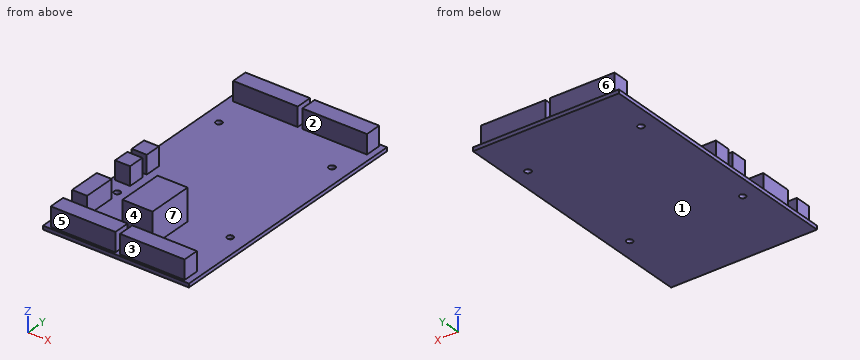
Autodesk Inventor part; units mm, degrees
ref_plane "YZ Plane" through (0, 0, 0) normal (1, 0, 0) x (0, 1, 0)
ref_plane "XZ Plane" through (0, 0, 0) normal (0, 1, 0) x (-1, 0, 0)
ref_plane "XY Plane" through (0, 0, 0) normal (0, 0, 1) x (1, 0, 0)
sketch "Sketch1" plane through (0, 0, 0) normal (0, 0, 1) x (1, 0, 0)
  line L0 (0, 0) -> (63.23, 0)
  line L1 (63.23, 0) -> (63.23, 113)
  line L2 (63.23, 113) -> (0, 113)
  line L3 (0, 113) -> (0, 0)
  line L4 (7.115, 91) -> (56.115, 91) construction
  line L5 (56.115, 91) -> (56.115, 33) construction
  line L6 (56.115, 33) -> (7.115, 33) construction
  line L7 (7.115, 33) -> (7.115, 91) construction
  circle A0 centre (7.115, 91) radius 1.35
  circle A1 centre (56.115, 91) radius 1.35
  circle A2 centre (56.115, 33) radius 1.35
  circle A3 centre (7.115, 33) radius 1.35
  point P0 (31.615, 91)
  point P1 (31.615, 113)
  dimension "d0" = 63.23
  dimension "d1" = 113
  dimension "d2" = 49
  dimension "d3" = 58
  dimension "d4" = 2.7
  dimension "d5" = 22
extrude "Extrusion1" add sketch "Sketch1" along normal blind 1.6
sketch "Sketch2" plane through (0, 0, 1.6) normal (0, 0, 1) x (1, 0, 0)
  point P0 (0, 0)
sketch "Sketch3" plane through (0, 0, 1.6) normal (0, 0, 1) x (1, 0, 0)
  line L0 (2.615, 112) -> (30.615, 112)
  line L1 (30.615, 112) -> (30.615, 105)
  line L2 (30.615, 105) -> (2.615, 105)
  line L3 (2.615, 105) -> (2.615, 112)
  line L4 (32.615, 112) -> (60.615, 112)
  line L5 (60.615, 112) -> (60.615, 105)
  line L6 (60.615, 105) -> (32.615, 105)
  line L7 (32.615, 105) -> (32.615, 112)
  line L8 (2.615, 1) -> (30.615, 1)
  line L9 (30.615, 1) -> (30.615, 8)
  line L10 (30.615, 8) -> (2.615, 8)
  line L11 (2.615, 8) -> (2.615, 1)
  line L12 (32.615, 1) -> (60.615, 1)
  line L13 (60.615, 1) -> (60.615, 8)
  line L14 (60.615, 8) -> (32.615, 8)
  line L15 (32.615, 8) -> (32.615, 1)
  line L16 (63.23, 113) -> (0, 113) construction
  line L17 (0, 0) -> (63.23, 0) construction
  line L18 (0, 113) -> (0, 0) construction
  dimension "d8" = 28
  dimension "d9" = 2
  dimension "d10" = 2
  dimension "d11" = 7
  dimension "d12" = 1
  dimension "d13" = 1
  dimension "d14" = 63.23
  dimension "d15" = 2.615
  dimension "d16" = 2.615
extrude "Extrusion2" add sketch "Sketch3" along normal blind 8.3
sketch "Sketch4" plane through (0, 0, 1.6) normal (0, 0, 1) x (1, 0, 0)
  line L0 (1.6, 28.5) -> (8.1, 28.5)
  line L1 (8.1, 28.5) -> (8.1, 14.5)
  line L2 (8.1, 14.5) -> (1.6, 14.5)
  line L3 (1.6, 14.5) -> (1.6, 28.5)
  line L4 (0, 0) -> (63.23, 0) construction
  line L5 (0, 113) -> (0, 0)
  line L6 (1.6, 55.5) -> (8.1, 55.5)
  line L7 (8.1, 55.5) -> (8.1, 48.5)
  line L8 (8.1, 48.5) -> (1.6, 48.5)
  line L9 (1.6, 48.5) -> (1.6, 55.5)
  line L10 (1.6, 46) -> (8.1, 46)
  line L11 (8.1, 46) -> (8.1, 39)
  line L12 (8.1, 39) -> (1.6, 39)
  line L13 (1.6, 39) -> (1.6, 46)
  dimension "d19" = 6.5
  dimension "d20" = 14
  dimension "d21" = 28.5
  dimension "d22" = 1.6
  dimension "d30" = 7
  dimension "d31" = 7
  dimension "d32" = 10.5
  dimension "d33" = 2.5
extrude "Extrusion3" add sketch "Sketch4" along normal blind 8
sketch "Sketch5" plane through (0, 0, 1.6) normal (0, 0, 1) x (1, 0, 0)
  line L0 (25.115, 32.3) -> (38.115, 32.3)
  line L1 (38.115, 32.3) -> (38.115, 12.3)
  line L2 (38.115, 12.3) -> (25.115, 12.3)
  line L3 (25.115, 12.3) -> (25.115, 32.3)
  line L4 (0, 0) -> (63.23, 0) construction
  point P0 (31.615, 12.3)
  point P1 (31.615, 0)
  dimension "d25" = 12.3
  dimension "d26" = 13
  dimension "d27" = 20
extrude "Extrusion4" add sketch "Sketch5" along normal blind 13.8
equation "\"d10\" = d9"
equation "\"d13\" = d12"
equation "\"d15\" = -0.5 * d9 + 0.5 * d14 - d8"
equation "\"d16\" = d15"
equation "\"d31\" = d30"
properties part number "PCB"
Part model, mm, in its own coordinate system. Face numbers are marked on the shaded views. A direction names the side the tool comes from. Round coordinates to 2 decimals unless told otherwise and drop trailing zeros. Write each loop counter-clockwise with the first axis right and the second up, starting at its lowest first coordinate (ties: lowest second). Pieces come first, ordered by that corner, then holes. Notation, with made-up numbers: M 22.25,86.25 L 56.25,86.25 A8 ccw 56.25,101.25 Z; hole C -32,64 d3. An arc over 180 degrees is marked long. Return JSON: item names as keys, results as strings. Group by question number.
(1) Saw through at C-C on x = 44.5. Write the cut outline in (y, z).
(2) Drill centre lines: probe 1 along Y at (x, z) = (33.5, 8); probe 2 along Y at (x, z) = (7.5, 5.5); probe 3 along X at (y, z) = (91, 0.85) (3 decimals). Where is each one in solid material? Low to high.
(3) Which spindle directions (+Z, -Z, +X, -X, +Y, -Y) get a long thin tool onto all of the face, cutting with end or side? Do the marked faces 4, 5, 6 and 7. Say none if no direction does.
(4) Saw through at B-B on y = 91. Write the cut outline in (x, z) (3 decimals), then the cut area to 3 significant figures.
(5) Saw through at D-D on z = 13.25. Write the cut outline in (x, y) (3 decimals), then the cut area to 3 significant figures.
(6) Pin check, flat tips, straight feed: pin 1 Ø3 at (x, y) = (7.5, 64) entering from +Z; pin 2 Ø6.5 at (x, z) = (18.5, 5.5) entering from -Y; pin 3 Ø7.5 at (x, y) = (46.5, 3) entering from +Z; pin 4 Ø4 at (x, y) = (9.5, 37) entering from -Z. Stop position of each tip, or through.
(7) Saw through at A-A on z = 4.5. Count the separate pieces of the cut face and the enclosed holes in it, then the cut area to 3 significant figures.
(8) Two-plate mould, pull along Y, no slides. Class the marked faces 1, 2 and 3: +Y half, -Y half, draft (parallel to the pull), parting line (faces both ways), or undercut.
Returned:
{
 "1": {"outline": "M 0,0 L 113,0 L 113,1.6 L 112,1.6 L 112,9.9 L 105,9.9 L 105,1.6 L 8,1.6 L 8,9.9 L 1,9.9 L 1,1.6 L 0,1.6 Z"},
 "2": {"probe 1": "1 to 8, 12.3 to 32.3, 105 to 112", "probe 2": "1 to 8, 14.5 to 28.5, 39 to 46, 48.5 to 55.5, 105 to 112", "probe 3": "0 to 5.765, 8.465 to 54.765, 57.465 to 63.23"},
 "3": {"face 4": "+Z, +X, -X", "face 5": "+Z, +X, -X, -Y", "face 6": "+Z, +X, -X, +Y", "face 7": "+Z, +X"},
 "4": {"outline": "M 0,0 L 5.765,0 L 5.765,1.6 L 0,1.6 Z; M 8.465,0 L 54.765,0 L 54.765,1.6 L 8.465,1.6 Z; M 57.465,0 L 63.23,0 L 63.23,1.6 L 57.465,1.6 Z", "area": "92.5 mm²"},
 "5": {"outline": "M 25.115,12.3 L 38.115,12.3 L 38.115,32.3 L 25.115,32.3 Z", "area": "260 mm²"},
 "6": {"pin 1": "z = 1.6", "pin 2": "y = 1", "pin 3": "z = 9.9", "pin 4": "z = 0"},
 "7": {"separate pieces": "8", "enclosed holes": "0", "area": "1,230 mm²"},
 "8": {"face 1": "draft", "face 2": "undercut", "face 3": "-Y half"}
}
